Could you check a few things on this model? Use its own coordinates, in mm. A direction names the side the tool comes from. Give positions to 0.01 mm unless a question says otherwise; leave off trailing zeros. Loops run counter-clockwise (first coordinate to the right, second up) from the corner with the lowest first, then second, coordinate; pieces in that order, holes last.
1. Imagine slicing it at D-D (z = 27.5). List the corners of the cut face in (x, y) for me.
2. Imagine slicing it at C-C (x = 29). List the corners of the cut face in (y, z) for me.
3. Thinking about a two-plate mould opening in X: for faces 1 (the cylindrical face through (38, -1.479, 71.506)), 2 (the cylindrical face through (59.74, -1.52, 64.99)), 3 (the flat face through (22, -2, 95)), which applies, +X half, -X half, draft (parallel to the pull), parting line (faces both ways), or undercut?
4. For faces 4 (the cylindrical face through (-1.48, 11.82, 8.68)), 5 (the flat face through (33, 0, 73)), 6 (the cylindrical face through (-1.48, 5.73, 29.74)), which set-ups out of +Z, -Z, +X, -X, +Y, -Y let a thin tool reach every point of the face, with its end or its side?
5. I need wall thicknesses on line 1 along Y through (x, z) = (-1, 7); line 2 along X through (y, z) = (53.5, 24). Which ranges of each line are inside material? Lowest first, please.
6. Imagine slicing it at B-B (z = 7.5). List the corners of the cut face in (x, y) for me.
7. For P1, Ø1.9, axis at x = 34.5, y = -0.5, coming from the -Z side; P2, Ø3, axis at x = 18.5, z = 75.5, coming from the +Y side; P3, Ø8, axis at y = 7, z = 17.5, coming from the +X side, each with a flat end and sliding along its axis, tell me the tip position at first contact or that it passes through.
8. Imagine slicing it at A-A (y = 17). List the corners of the cut face in (x, z) for me.
```python
from build123d import *

# Parameters (mm, degrees)
SM_BASE_FLANGE_1_DEPTH = 95
FILLET_1_R             = 17.5
SKETCH_9_R             = 2.15
SKETCH_9_R_2           = 1.6
CUT_EXTRUDE_1_DEPTH    = 10
FILLET_2_R             = 5
CUT_EXTRUDE_START      = -10
CUT_EXTRUDE_2_DEPTH    = 10
SKETCH_14_W            = 71.334593732
SKETCH_14_H            = 13.225299836
CUT_EXTRUDE_3_DEPTH    = 60
FILLET_4_R             = 17.5
FILLET_5_R             = 17.5
SKETCH_15_R            = 6
CUT_EXTRUDE_4_DEPTH    = 10
SKETCH_16_R            = 1.25
CUT_EXTRUDE_5_DEPTH    = 10


# Sheet-metal steps are written as plain solids
with BuildPart() as part:
    # Sketch 2 → 基材-凸緣1 (new body)
    with BuildSketch(Plane.XY):
        with BuildLine():
            Line((65, 0), (0.7366, 0))
            ThreePointArc((0.7366, 0), (0.215745145, 0.215745145), (0, 0.7366))
            Line((0, 0.7366), (0, 95))
            Line((0, 95), (-3, 95))
            Line((-3, 95), (-3, 0.7366))
            ThreePointArc((-3, 0.7366), (-1.905575199, -1.905575199), (0.7366, -3))
            Line((0.7366, -3), (65, -3))
            Line((65, -3), (65, 0))
        make_face()
    extrude(amount=SM_BASE_FLANGE_1_DEPTH)

    # 圓角1
    fillet_1_edges = [part.edges().sort_by_distance(p)[0] for p in [
        (65, -1.5, 95),
        (65, -1.5, 0),
    ]]
    fillet(fillet_1_edges, radius=FILLET_1_R)

    # 草圖9 → 除料-伸長1 (cut)
    with BuildSketch(Plane(origin=(0, 0, 0), x_dir=(0, 0, -1), z_dir=(1, 0, 0))):
        with Locations((-7.5, 60.2366)):
            Circle(SKETCH_9_R)
        with Locations((-27.5, 60.2366)):
            Circle(SKETCH_9_R)
        with BuildLine():
            ThreePointArc((-5.35, 84.2366), (-7.5, 86.3866), (-9.65, 84.2366))
            ThreePointArc((-9.65, 84.2366), (-7.5, 82.0866), (-5.35, 84.2366))
        make_face()
        with Locations((-27.5, 84.2366)):
            Circle(SKETCH_9_R)
        with Locations((-7.5, 30.7366)):
            Circle(SKETCH_9_R_2)
        with Locations((-7.5, 10.7366)):
            Circle(SKETCH_9_R_2)
        with Locations((-27.5, 10.7366)):
            Circle(SKETCH_9_R_2)
        with Locations((-27.5, 30.7366)):
            Circle(SKETCH_9_R_2)
    extrude(amount=-CUT_EXTRUDE_1_DEPTH, mode=Mode.SUBTRACT)

    # 圓角2
    fillet_2_edges = [part.edges().sort_by_distance(p)[0] for p in [
        (-1.5, 95, 95),
        (-1.5, 95, 0),
    ]]
    fillet(fillet_2_edges, radius=FILLET_2_R)

    # 草圖12 → 除料-伸長2 (cut)
    with BuildSketch(Plane(origin=(0, 0, 0), x_dir=(0, 0, -1), z_dir=(1, 0, 0)).offset(CUT_EXTRUDE_START)):
        Polygon((-35, 0.7366), (-35, 60), (-60, 0.7366), align=None)
        with BuildLine():
            Line((-90, 95), (-35, 95))
            Line((-35, 95), (-95, 0.7366))
            Line((-95, 0.7366), (-95, 90))
            ThreePointArc((-95, 90), (-93.535533906, 93.535533906), (-90, 95))
        make_face()
    extrude(amount=CUT_EXTRUDE_2_DEPTH, mode=Mode.SUBTRACT)

    # 草圖14 → 除料-伸長3 (cut)
    with BuildSketch(Plane(origin=(0, 0, 0), x_dir=(-1, 0, 0), z_dir=(0, 0, -1))):
        with Locations((-32.667296866, -5.876049918)):
            Rectangle(SKETCH_14_W, SKETCH_14_H)
    extrude(amount=-CUT_EXTRUDE_3_DEPTH, mode=Mode.SUBTRACT)

    # 圓角4
    fillet_4_edges = [part.edges().sort_by_distance(p)[0] for p in [
        (-1.5, 0.7366, 35),
        (-1.5, 0.7366, 0),
        (65, -1.5, 60),
    ]]
    fillet(fillet_4_edges, radius=FILLET_4_R - 0.0001)  # a hair under: the kernel refuses the full size

    # 圓角5
    fillet_5_edges = [part.edges().sort_by_distance(p)[0] for p in [
        (-1.5, 95, 35),
    ]]
    fillet(fillet_5_edges, radius=FILLET_5_R)

    # 草圖15 → 除料-伸長4 (cut)
    with BuildSketch(Plane(origin=(0, 0, 0), x_dir=(1, 0, 0), z_dir=(0, 1, 0))):
        with Locations(Location((37.7366, -77.5, 0), (0, 0, 270))):
            Circle(SKETCH_15_R)
    extrude(amount=-CUT_EXTRUDE_4_DEPTH, mode=Mode.SUBTRACT)

    # 草圖16 → 除料-伸長5 (cut)
    with BuildSketch(Plane(origin=(0, 0, 0), x_dir=(1, 0, 0), z_dir=(0, 1, 0))):
        with Locations(Location((6.2466, -72.5, 0), (0, 0, 270))):
            Circle(SKETCH_16_R)
        with Locations(Location((55.7466, -72.5, 0), (0, 0, 270))):
            Circle(SKETCH_16_R)
        with Locations(Location((55.7466, -82.5, 0), (0, 0, 270))):
            Circle(SKETCH_16_R)
        with Locations(Location((6.2466, -82.5, 0), (0, 0, 270))):
            Circle(SKETCH_16_R)
    extrude(amount=-CUT_EXTRUDE_5_DEPTH, mode=Mode.SUBTRACT)


solid = part.part
```
Derived:
1. outline: (-3, 3.88) - (0, 3.88) - (0, 9.14) - (-3, 9.14) - close; (-3, 12.34) - (0, 12.34) - (0, 29.14) - (-3, 29.14) - close; (-3, 32.34) - (0, 32.34) - (0, 58.09) - (-3, 58.09) - close; (-3, 62.39) - (0, 62.39) - (0, 82.09) - (-3, 82.09) - close; (-3, 86.39) - (0, 86.39) - (0, 94.87) - (-3, 94.87) - close
2. outline: (-3, 60) - (0, 60) - (0, 95) - (-3, 95) - close
3. face 1: undercut
3. face 2: +X half
3. face 3: draft
4. face 4: +X, -X
4. face 5: +Z, -Z, +X, +Y
4. face 6: +X, -X, -Y
5. line 1: y = 4.24 to 9.22, 12.26 to 29.22, 32.26 to 58.15, 62.33 to 82.15, 86.33 to 95
5. line 2: x = -3 to 0
6. outline: (-3, 3.88) - (0, 3.88) - (0, 9.14) - (-3, 9.14) - close; (-3, 12.34) - (0, 12.34) - (0, 29.14) - (-3, 29.14) - close; (-3, 32.34) - (0, 32.34) - (0, 58.09) - (-3, 58.09) - close; (-3, 62.39) - (0, 62.39) - (0, 82.09) - (-3, 82.09) - close; (-3, 86.39) - (0, 86.39) - (0, 95) - (-3, 95) - close
7. P1: stops at z = 60
7. P2: stops at y = 0
7. P3: stops at x = 0
8. outline: (-3, 0.04) - (0, 0.04) - (0, 34.96) - (-3, 34.96) - close; (-3, 53.14) - (0, 53.14) - (0, 84.65) - (-3, 84.65) - close
